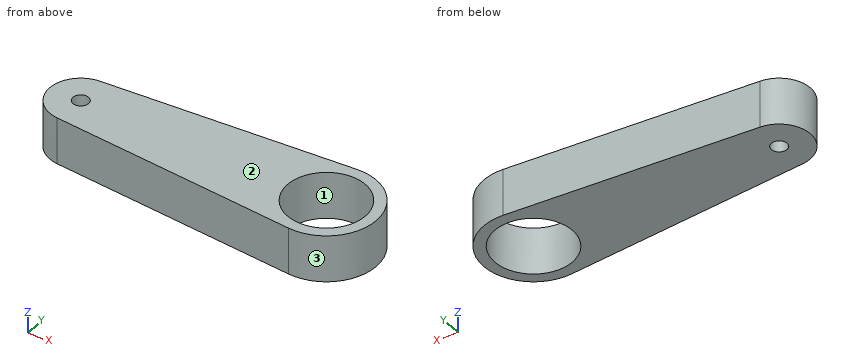
from build123d import *

# Parameters (mm, degrees)
CROQUIS2_R              = 2.5
CROQUIS2_R_2            = 0.5
SALIENTE_EXTRUIR1_DEPTH = 1.5


with BuildPart() as part:
    # Croquis2 → Saliente-Extruir1 (new, symmetric)
    with BuildSketch(Plane.XY):
        with BuildLine():
            ThreePointArc((-0.152380952, 1.994186562), (-2, 0), (-0.152380952, -1.994186562))
            Line((-0.152380952, -1.994186562), (15.506190476, -3.1906985))
            ThreePointArc((15.506190476, -3.1906985), (18.95, 0), (15.506190476, 3.1906985))
            Line((15.506190476, 3.1906985), (-0.152380952, 1.994186562))
        make_face()
        with Locations((15.75, 0)):
            Circle(CROQUIS2_R, mode=Mode.SUBTRACT)
        Circle(CROQUIS2_R_2, mode=Mode.SUBTRACT)
    extrude(amount=SALIENTE_EXTRUIR1_DEPTH, both=True)


solid = part.part
Check sheet for the modelled part. Datum: model origin and axes. Units: mm. Face numbers are marked on the shaded views. Round coordinates to 2 decimals unless told otherwise and drop trailing zeros. Loops run counter-clockwise (first coordinate to the right, second up) from the corner with the lowest first, then second, coordinate; pieces in that order, holes last.
1. Gauge pin test, flat ends, axial feed: pin 1 Ø1 at (x, z) = (4, 0.5) entering from +Y; pin 2 Ø1.5 at (y, z) = (2, 0.5) entering from -X. Record the tip position at first contact, or that the pin passes through.
2. Sectioned sample at A-A on y = 0. Record the boundary of the cut face in (x, z).
3. Mould release check, pull along Y, two halves, no side actions. Record for the marked faces 1, 2 and 3: released by +Y, released by -Y, zero draft, split by the parting line, or undercut.
4. Sectioned sample at B-B on x = 15.75. Record the boundary of the cut face in (y, z), and give its area (3 significant figures).
5. Sectioned sample at C-C on y = 1.25. Record the boundary of the cut face in (x, z), and give its area (3 significant figures).
6. Scan lines: probe 1 along X at (y, z) = (-0.25, -1.05); probe 2 along Y at (x, z) = (15.75, -0.4); probe 3 along Y at (x, z) = (15.25, 0.95). Record each from-to range of solid material in increasing order.
7. Sectioned sample at D-D on z = -0.4. Record the boundary of the cut face in (x, y), and give its area (3 significant figures).
Recorded:
1. pin 1: stops at y = 2.35
1. pin 2: stops at x = -1.56
2. outline: (-2, -1.5) - (-0.5, -1.5) - (-0.5, 1.5) - (-2, 1.5) - close; (0.5, -1.5) - (13.25, -1.5) - (13.25, 1.5) - (0.5, 1.5) - close; (18.25, -1.5) - (18.95, -1.5) - (18.95, 1.5) - (18.25, 1.5) - close
3. face 1: undercut
3. face 2: zero draft
3. face 3: split by the parting line
4. outline: (-3.2, -1.5) - (-2.5, -1.5) - (-2.5, 1.5) - (-3.2, 1.5) - close; (2.5, -1.5) - (3.2, -1.5) - (3.2, 1.5) - (2.5, 1.5) - close
4. area: 4.20 mm2
5. outline: (-1.56, -1.5) - (13.58, -1.5) - (13.58, 1.5) - (-1.56, 1.5) - close; (17.92, -1.5) - (18.7, -1.5) - (18.7, 1.5) - (17.92, 1.5) - close
5. area: 47.8 mm2
6. probe 1: x = -1.98 to -0.43, 0.43 to 13.26, 18.24 to 18.94
6. probe 2: y = -3.2 to -2.5, 2.5 to 3.2
6. probe 3: y = -3.17 to -2.45, 2.45 to 3.17
7. outline: (-0.15, -1.99) - (15.51, -3.19) arc R3.2 ccw (long way) to (15.51, 3.19) - (-0.15, 1.99) arc R2 ccw to start; hole circle Ø1 at (0, 0); hole circle Ø5 at (15.75, 0)
7. area: 84.1 mm2
